from build123d import *

# Parameters (mm, degrees)
F2_SIZE2 = 11.4300523028
F2_SIZE  = 1
F3_SIZE  = 1


# Not quite as in the source:
# - a fillet or chamfer that OpenCascade refuses, or shapes differently, is made with other operations: its cross-section is extruded or revolved along the edge and cut away or added


with BuildPart() as f1:
    # F0 (on Front) → F1 (revolve)
    with BuildSketch(Plane.XZ):
        Polygon((-14.5, 15), (-16.5, 15), (-16.5, 0), (-10, -6.5), (-10, -17), (-8, -17), (-8, -5.6715728753), (-14.5, 0.8284271247), align=None)
    revolve(axis=Axis((0, 0, 0.14814813), (0, 0, -1)))

    # F2
    f2_edges = [f1.edges().sort_by_distance(p)[0] for p in [
        (16.5, 0, 15),
    ]]
    chamfer(f2_edges, length=F2_SIZE, length2=F2_SIZE2)

    # F3
    f3_edges = [f1.edges().sort_by_distance(p)[0] for p in [
        (10, 0, -17),
    ]]
    chamfer(f3_edges, length=F3_SIZE)

    # F4: chamfer of 1 x 11.4300523028 on 1 edges, made by hand

    # F4_s1 → F4_t2 (revolve, cut)
    with BuildSketch(Plane.XZ):
        Polygon((-9, -17), (-8, -5.5699476972), (-8, -17), align=None)
    revolve(axis=Axis((0, 0, -17), (0, 0, -1)), mode=Mode.SUBTRACT)


solid = f1.part
Verification items for the finished model (mm, model axes). A direction names the side the tool comes from. Coordinates: 2 decimals unless noted, no trailing zeros. Order: outer loops, then holes, each group sorted by start corner. A loop starts at its lowest first (then second) coordinate and runs counter-clockwise, first axis right, second up.
1. Go/stop test with flat-tipped pins: pin 1 Ø5 at (x, y) = (-13, 3) entering from -Z; pin 2 Ø5 at (x, z) = (7.5, -13.5) entering from +Y; pin 3 Ø6 at (y, z) = (11.5, -6) entering from -X. Record where each tip stops, or that it passes through.
Results found:
pin 1: stops at z = -5.66
pin 2: stops at y = 8.66
pin 3: stops at x = -8.5
2. Sectioned sample at C-C, the plane z = 10. Record the cut outline in (x, y), and give its area (3 significant figures).
Results found:
outline: circle Ø31.87 at (0, 0); hole circle Ø29 at (0, 0)
area: 137 mm2
3. Release check for a two-part mould opening along Y. For faces 3 (the face through (6, -14, 15)), 4 (the face through (1.092, 8.316, -9.993)), 5 (the face through (-15.24, -6.32, 1.76)) record: +Y half, -Y half, draft (parallel to the pull), parting line (faces both ways), or undercut.
Results found:
face 3: draft
face 4: undercut
face 5: parting line
4. Sectioned sample at A-A, the plane y = 0. Record the cut outline in (x, z).
Results found:
outline: (-16.5, 0) - (-10, -6.5) - (-10, -16) - (-9, -17) - (-8.01, -5.66) - (-14.5, 0.83) - (-14.5, 15) - (-15.5, 15) - (-16.5, 3.57) - close; (8.01, -5.66) - (9, -17) - (10, -16) - (10, -6.5) - (16.5, 0) - (16.5, 3.57) - (15.5, 15) - (14.5, 15) - (14.5, 0.83) - close
5. Scan lines: line 1 (Y direction, x = 5, z = -1.5); line 2 (Y direction, x = 0, z = 11.25); line 3 (X direction, y = -6, z = -6.5). Record each from-to range of solid material in increasing order.
Results found:
line 1: y = -14.14 to -11.1, 11.1 to 14.14
line 2: y = -15.83 to -14.5, 14.5 to 15.83
line 3: x = -8 to -5.41, 5.41 to 8
6. Set-up check for faces 1 (the face through (2.17, -9.76, -11.32)), 2 (the face through (-6.691, -12.864, 8.013)): record each of +Z, -Z, +X, -X, +Y, -Y from which the full face is reachable in a straight line by a thin tool's end or side.
Results found:
face 1: -Z
face 2: +Z
